from build123d import *

# Parameters (mm, degrees)
F0_W     = 83.0704942346
F0_H     = 31.7708207294
F1_DEPTH = 19.05
F3_DEPTH = 35.052
F4_W     = 83.0704942346
F4_H     = 7.5783608481
F5_DEPTH = 25.4
F7_DEPTH = 25.4
F8_R     = 5.7653950386
F9_DEPTH = 25.4


with BuildPart() as f1:
    # F0 (on Front) → F1 (new body)
    with BuildSketch(Plane.XZ):
        with Locations((-2.4775415659, 27.3986891843)):
            Rectangle(F0_W, F0_H)
    extrude(amount=-F1_DEPTH)

    # F2 (on face) → F3 (cut)
    with BuildSketch(Plane(origin=(0, 0, 11.5132788196), x_dir=(1, 0, 0), z_dir=(0, 0, -1))):
        Polygon((-31.7708216608, -10.9303286299), (-24.4839340448, -19.05), (16.6140999645, -19.05), (24.775410071, -10.9303286299), align=None)
    extrude(amount=-F3_DEPTH, mode=Mode.SUBTRACT)

    # F4 (on face) → F5 (join)
    with BuildSketch(Plane.XZ):
        with Locations((-2.4775415659, 15.3024592437)):
            Rectangle(F4_W, F4_H)
    extrude(amount=F5_DEPTH)

    # F6 (on face) → F7 (cut)
    with BuildSketch(Plane.XY.offset(19.0916396677)):
        Polygon((39.0577055514, -25.4), (39.0577055514, -12.7), (23.9009838551, -25.4), align=None)
        Polygon((-44.0127886832, -25.4), (-28.8560669869, -25.4), (-44.0127886832, -12.7), align=None)
    extrude(amount=-F7_DEPTH, mode=Mode.SUBTRACT)

    # F8 (on face) → F9 (cut)
    with BuildSketch(Plane.XZ):
        with Locations((0, 31.1878696084)):
            Circle(F8_R)
    extrude(amount=-F9_DEPTH, mode=Mode.SUBTRACT)


solid = f1.part
Design review of the part built by this model. Coordinates are the model's own, in mm. A direction names the side the tool comes from. Round coordinates to 2 decimals unless told otherwise and drop trailing zeros. Write each loop counter-clockwise with the first axis right and the second up, starting at its lowest first coordinate (ties: lowest second). Pieces come first, ordered by that corner, then holes.
Item 1: Consider section A-A on x = 0. Give the boundary of the cut face in (y, z), and give its area (3 significant figures).
Item 2: For faces 1 (the flat face through (-3, 0, 26)), 2 (the flat face through (-44.013, 7, 24)), 3 (the flat face through (-3, 10.93, 24)), list the 3-axis set-ups (+Z, -Z, +X, -X, +Y, -Y) from which the entire face can be reached by the end or side of a thin tool; tool diameter is ignored.
Item 3: Consider section C-C on z = 32. Give the boundary of the cut face in (x, y), and give its area (3 significant figures).
Item 4: Draft analysis for pull direction Y (two halves, no side actions). For faces 4 (the flat face through (20.638, 15.047, 27.176)), 5 (the flat face through (-3, -3, 11.513)), 6 (the flat face through (31.585, -18.961, 15.356)), state which applies: released by +Y, released by -Y, zero draft, split by the parting line, or undercut.
Item 5: Consider section D-D on y = 6. Give the boundary of the cut face in (x, z), and give its area (3 significant figures).
Item 6: Wall thickness on L1, parallel to Z at x = 0, y = 4; L2, parallel to X at y = 3, z = 31; L3, parallel to Z at x = 4, y = -0.5: over which ranges is each line inside the solid? List them lowest first.
Item 7: Consider section B-B on z = 23. Give the boundary of the cut face in (x, y).
Item 8: For pin 1 Ø8 at (x, y) = (19.5, -18) entering from +Z; pin 2 Ø1 at (x, z) = (2, 27.5) entering from -Y; pin 3 Ø7.5 at (x, z) = (14.5, 32) entering from -Y; pin 4 Ø2 at (x, z) = (5.5, 18) entering from +Y, all flat-tipped, find the tip position at first contact; note any pin that passes through.
Check values:
1. outline: (-25.4, 11.51) - (10.93, 11.51) - (10.93, 25.42) - (0, 25.42) - (0, 19.09) - (-25.4, 19.09) - close; (0, 36.95) - (10.93, 36.95) - (10.93, 43.28) - (0, 43.28) - close
1. area: 414 mm2
2. face 1: +Z, +X, -X, -Y
2. face 2: +Z, -Z, -X, +Y, -Y
2. face 3: +Z, -Z
3. outline: (-44.01, 0) - (-5.71, 0) - (-5.71, 10.93) - (-31.77, 10.93) - (-24.48, 19.05) - (-44.01, 19.05) - close; (5.71, 0) - (39.06, 0) - (39.06, 19.05) - (16.61, 19.05) - (24.78, 10.93) - (5.71, 10.93) - close
3. area: 1,060 mm2
4. face 4: undercut
4. face 5: zero draft
4. face 6: released by -Y
5. outline: (-44.01, 11.51) - (39.06, 11.51) - (39.06, 43.28) - (-44.01, 43.28) - close; hole circle Ø11.53 at (0, 31.19)
5. area: 2,530 mm2
6. L1: z = 11.51 to 25.42, 36.95 to 43.28
6. L2: x = -44.01 to -5.76, 5.76 to 39.06
6. L3: z = 11.51 to 19.09
7. outline: (-44.01, 0) - (39.06, 0) - (39.06, 19.05) - (16.61, 19.05) - (24.78, 10.93) - (-31.77, 10.93) - (-24.48, 19.05) - (-44.01, 19.05) - close
8. pin 1: stops at z = 19.09
8. pin 2: passes through
8. pin 3: stops at y = 0
8. pin 4: stops at y = 10.93
